Autodesk Inventor part; units mm, degrees
ref_plane "YZ Plane" through (0, 0, 0) normal (1, 0, 0) x (0, 1, 0)
ref_plane "XZ Plane" through (0, 0, 0) normal (0, 1, 0) x (-1, 0, 0)
ref_plane "XY Plane" through (0, 0, 0) normal (0, 0, 1) x (1, 0, 0)
sketch "Esboço1" plane through (0, 0, 0) normal (0, 0, 1) x (1, 0, 0)
  circle A0 centre (0, 0) radius 12.5
  circle A1 centre (0, 0) radius 2
  dimension "d0" = 25
  dimension "d1" = 4
extrude "Extrusão1" add sketch "Esboço1" against normal blind 12
sketch "Esboço2" plane through (0, 0, 0) normal (0, 0, 1) x (1, 0, 0)
  point P0 (0, 0)
fillet "Arredondamento1" radius 0.5 1 edges at (-12.5, 0, 0)
sketch "Esboço3" plane through (0, 0, 0) normal (0, 0, 1) x (1, 0, 0)
  circle A0 centre (0, 10.5) radius 1.5
  circle A1 centre (0, 0) radius 12
  dimension "d5" = 3
extrude "Extrusão2" cut sketch "Esboço3" against normal blind 12 contours A0
properties part number "crank_wheel" material "Aluminum 6061-AHC"
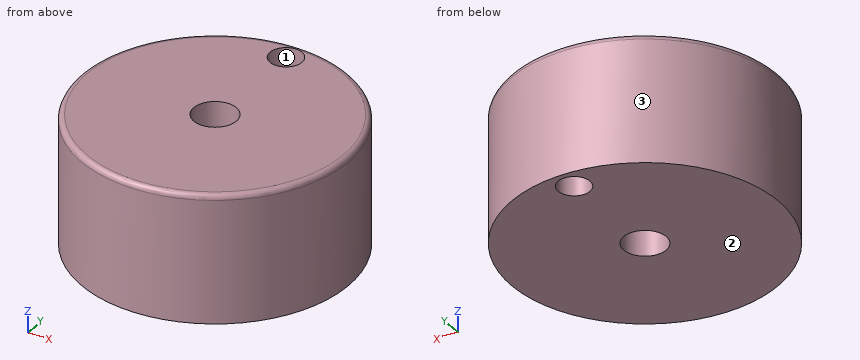
Here's how the part is built. I have some questions about the finished solid (model axes, mm). Face numbers are marked on the shaded views. Coordinates: 2 decimals unless noted, no trailing zeros. Order: outer loops, then holes, each group sorted by start corner. A loop starts at its lowest first (then second) coordinate and runs counter-clockwise, first axis right, second up. Notation, with made-up numbers: (-11, 20.5) -> (46, 20.5) arc R15 ccw to (46, 34.5) -> close; hole circle Ø6 at (73, 87.25). An arc over 180 degrees is marked (long way). Return JSON: item names as keys, results as strings.
1) I'm going to push flat-ended pins straight in: P1, Ø5, axis at x = -9, z = -9.5, coming from the -Y side; P2, Ø4, axis at x = -7.5, z = -4.5, coming from the -Y side (3 decimals); P3, Ø2.5, axis at x = 0, y = 10.5, coming from the -Z side. Where does each tip first touch, or does it pass through?
Conclusion:
{"P1": "stops at y = -10.68", "P2": "stops at y = -11.225", "P3": "passes through"}
2) Thinking about a two-plate mould opening in X: for the marked faces 1, 2 and 3, which applies, +X half, -X half, draft (parallel to the pull), parting line (faces both ways), or undercut?
Conclusion:
{"face 1": "undercut", "face 2": "draft", "face 3": "parting line"}
3) If I drill on probe 1 along Y at (x, z) = (0, -9); probe 2 along Y at (x, z) = (-0.75, -4.25); probe 3 along X at (y, z) = (-1.5, -7.5), over which ranges is the centre line in solid material (lowest first)?
Conclusion:
{"probe 1": "y = -12.5 to -2, 2 to 9, 12 to 12.5", "probe 2": "y = -12.48 to -1.85, 1.85 to 9.2, 11.8 to 12.48", "probe 3": "x = -12.41 to -1.32, 1.32 to 12.41"}
4) If we section it at A-A on y = 0: List the corners of the cut face in (x, z) for me.
Conclusion:
{"outline": "(-12.5, -12) -> (-2, -12) -> (-2, 0) -> (-12, 0) arc R0.5 ccw to (-12.5, -0.5) -> close; (2, -12) -> (12.5, -12) -> (12.5, -0.5) arc R0.5 ccw to (12, 0) -> (2, 0) -> close"}
5) If we section it at B-B on z = -9.25: List the corners of the cut face in (x, y) for me, plus the area to 3 significant figures.
Conclusion:
{"outline": "circle Ø25 at (0, 0); hole circle Ø4 at (0, 0); hole circle Ø3 at (0, 10.5)", "area": "471 mm²"}
